from build123d import *

# Parameters (mm, degrees)
SKETCH_W      = 100
SKETCH_H      = 15.25
SKETCH_R      = 1.75
PAD_DEPTH     = 3
SKETCH001_W   = 100
SKETCH001_H   = 5
PAD001_DEPTH  = 10
SKETCH002_R   = 3.5
SKETCH002_R_2 = 1.75
PAD002_DEPTH  = 5
SKETCH003_W   = 6.062178
SKETCH003_H   = 8.25
PAD003_DEPTH  = 5
CHAMFER_SIZE  = 5


with BuildPart() as part:
    # Sketch → Pad (new body)
    with BuildSketch(Plane.XY):
        with Locations((0, -7.625)):
            Rectangle(SKETCH_W, SKETCH_H)
        with Locations((-40, -10)):
            Circle(SKETCH_R, mode=Mode.SUBTRACT)
        with Locations((40, -10)):
            Circle(SKETCH_R, mode=Mode.SUBTRACT)
    extrude(amount=PAD_DEPTH)

    # Sketch001 (on Face7 of Pad) → Pad001 (join)
    with BuildSketch(Plane(origin=(0, 0, 0), x_dir=(1, 0, 0), z_dir=(0, 0, -1))):
        with Locations((0, 2.5)):
            Rectangle(SKETCH001_W, SKETCH001_H)
    extrude(amount=PAD001_DEPTH)

    # Sketch002 (on Face5 of Pad001) → Pad002 (join)
    with BuildSketch(Plane.XY.offset(3)):
        with Locations((-40, -10)):
            Circle(SKETCH002_R)
        with Locations((-40, -10)):
            Circle(SKETCH002_R_2, mode=Mode.SUBTRACT)
        with Locations((40, -10)):
            Circle(SKETCH002_R)
        with Locations((40, -10)):
            Circle(SKETCH002_R_2, mode=Mode.SUBTRACT)
    extrude(amount=PAD002_DEPTH)

    # Sketch003 (on Face17 of Pad002) → Pad003 (join)
    with BuildSketch(Plane.XY.offset(8)):
        with Locations((-40, -4.125)):
            Rectangle(SKETCH003_W, SKETCH003_H)
        with Locations((40, -4.125)):
            Rectangle(SKETCH003_W, SKETCH003_H)
    extrude(amount=-PAD003_DEPTH)

    # Chamfer
    chamfer_edges = [part.edges().sort_by_distance(p)[0] for p in [
        (-40, 0, 8),
        (40, 0, 8),
    ]]
    chamfer(chamfer_edges, length=CHAMFER_SIZE)


solid = part.part
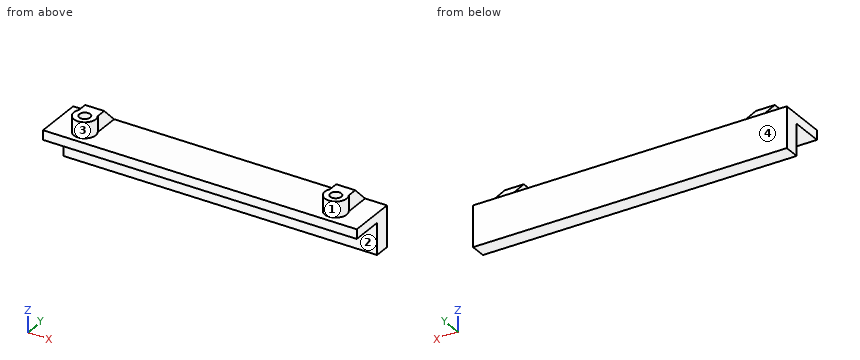
Check sheet for the modelled part. Datum: model origin and axes. Units: mm. Face numbers are marked on the shaded views. A direction names the side the tool comes from. Round coordinates to 2 decimals unless told otherwise and drop trailing zeros. Order: outer loops, then holes, each group sorted by start corner. A loop starts at its lowest first (then second) coordinate and runs counter-clockwise, first axis right, second up.
Q1. Cross-section at A-A, the plane z = 4.25. Enter the section's corners in (x, y), plus the area to 3 significant figures.
Filled sheet:
outline: (-43.03, -8.25) arc R3.5 ccw (long way) to (-36.97, -8.25) - (-36.97, -1.25) - (-43.03, -1.25) - close; (36.97, -8.25) arc R3.5 ccw (long way) to (43.03, -8.25) - (43.03, -1.25) - (36.97, -1.25) - close; hole circle Ø3.5 at (-40, -10); hole circle Ø3.5 at (40, -10)
area: 128 mm2
Q2. Draft check along X on the marked faces 1 and 2. Enter one of: pulls with the +X half, pulls with the -X half, needs draft (parallel to the pull), parting line crosses it, or undercut.
Filled sheet:
face 1: undercut
face 2: needs draft
Q3. Set-up check for the marked faces 3 and 4: record each of +Z, -Z, +X, -X, +Y, -Y from which the full face is reachable in a straight line by a thin tool's end or side.
Filled sheet:
face 3: +Z
face 4: +Z, -Z, +X, -X, +Y
Q4. Scan lines: L1, parallel to X at y = -10, z = 2; L2, parallel to X at y = -10, z = 5.25; L3, parallel to X at y = -5, z = 3.25. Record each from-to range of solid material in increasing order.
Filled sheet:
L1: x = -50 to -41.75, -38.25 to 38.25, 41.75 to 50
L2: x = -43.5 to -41.75, -38.25 to -36.5, 36.5 to 38.25, 41.75 to 43.5
L3: x = -43.03 to -36.97, 36.97 to 43.03
Q5. Cross-section at B-B, the plane x = 40. Enter the section's corners in (y, z).
Filled sheet:
outline: (-15.25, 0) - (-11.75, 0) - (-11.75, 8) - (-13.5, 8) - (-13.5, 3) - (-15.25, 3) - close; (-8.25, 0) - (-5, 0) - (-5, -10) - (0, -10) - (0, 3) - (-5, 8) - (-8.25, 8) - close
Q6. Cross-section at C-C, the plane y = -10. Enter the section's corners in (x, z), plus the area to 3 significant figures.
Filled sheet:
outline: (-50, 0) - (-41.75, 0) - (-41.75, 8) - (-43.5, 8) - (-43.5, 3) - (-50, 3) - close; (-38.25, 0) - (38.25, 0) - (38.25, 8) - (36.5, 8) - (36.5, 3) - (-36.5, 3) - (-36.5, 8) - (-38.25, 8) - close; (41.75, 0) - (50, 0) - (50, 3) - (43.5, 3) - (43.5, 8) - (41.75, 8) - close
area: 314 mm2
Q7. Cross-section at D-D, the plane y = -6. Enter the section's corners in (x, z).
Filled sheet:
outline: (-50, 0) - (50, 0) - (50, 3) - (43.03, 3) - (43.03, 8) - (36.97, 8) - (36.97, 3) - (-36.97, 3) - (-36.97, 8) - (-43.03, 8) - (-43.03, 3) - (-50, 3) - close
Q8. Depth check by flat-ended pin: P1, Ø10, axis at x = 17, z = 5, coming from the +Y side; P2, Ø2.5, axis at y = -3.5, z = 5.5, coming from the -X side; P3, Ø4, axis at y = -5.5, z = 6.5, coming from the +X side. Enter the tip coordinate at first touch or a pass-through.
Filled sheet:
P1: stops at y = 0
P2: stops at x = -43.03
P3: stops at x = 43.03
